Here's how the part is built. I have some questions about the finished solid (model axes, mm). A direction names the side the tool comes from. Coordinates: 2 decimals unless noted, no trailing zeros. Order: outer loops, then holes, each group sorted by start corner. A loop starts at its lowest first (then second) coordinate and runs counter-clockwise, first axis right, second up.
```python
from build123d import *

# Parameters (mm, degrees)
BOSS_EXTRUDE1_DEPTH = 6.35


with BuildPart() as part:
    # Sketch2 → Boss-Extrude1 (new body)
    with BuildSketch(Plane(origin=(0, 0, 0), x_dir=(1, 0, 0), z_dir=(0, 1, 0))):
        with BuildLine():
            Line((-50.75013925, 9.494238665), (-40.191557527, 3.398238665))
            Line((-40.191557527, 3.398238665), (-50.75013925, -2.697761335))
            Line((-50.75013925, -2.697761335), (-40.191557527, -8.793761335))
            Line((-40.191557527, -8.793761335), (-50.75013925, -14.889761335))
            Line((-50.75013925, -14.889761335), (-64.40263925, -14.889761335))
            ThreePointArc((-64.40263925, -14.889761335), (-65.584061474, -2.697761335), (-64.40263925, 9.494238665))
            Line((-64.40263925, 9.494238665), (-50.75013925, 9.494238665))
        make_face()
    extrude(amount=BOSS_EXTRUDE1_DEPTH)


solid = part.part
```
Q1. For faces 1 (the flat face through (-45.545, 3.131, 5.703)), 2 (the flat face through (-45.545, 3.131, -6.489)), which set-ups out of +Z, -Z, +X, -X, +Y, -Y let a thin tool reach every point of the face, with its end or its side?
Q2. If we section it at B-B on y = 4.5: Write out the boundary of the cut face in (x, z).
Q3. If we section it at D-D on z = 3.5: Write out the boundary of the cut face in (x, y).
Q4. We'd pull the mould along Z, two halves only. Please class faces 3 (the flat face through (-45.4, 3.13, -0.39)), 4 (the flat face through (-56, 6.35, 3)), 5 (the flat face through (-58, 3, -9.494)): pulls with the +Z half, pulls with the -Z half, needs draft (parallel to the pull), parting line crosses it, or undercut.
Q5. If we section it at A-A on x = -47: Write out the boundary of the cut face in (y, z).
Q6. I need wall thicknesses on L1, parallel to Z at x = -46, y = 2.5; L2, parallel to Z at x = -43.75, y = 1.75; L3, parallel to X at y = 2.25, z = 12.5. Which ranges of each line are inside material? Lowest first, please.
Q7. If we section it at C-C on x = -43.25: Write out the boundary of the cut face in (y, z).
Reply:
1. face 1: +X, +Y, -Y
1. face 2: -Z, +X, +Y, -Y
2. outline: (-64.4, -9.49) - (-50.75, -9.49) - (-40.19, -3.4) - (-50.75, 2.7) - (-40.19, 8.79) - (-50.75, 14.89) - (-64.4, 14.89) arc R63.5 ccw to start
3. outline: (-65.58, 0) - (-49.36, 0) - (-49.36, 6.35) - (-65.58, 6.35) - close
4. face 3: undercut
4. face 4: needs draft
4. face 5: pulls with the -Z half
5. outline: (0, -7.33) - (6.35, -7.33) - (6.35, 0.53) - (0, 0.53) - close; (0, 4.86) - (6.35, 4.86) - (6.35, 12.72) - (0, 12.72) - close
6. L1: z = -6.75 to -0.04, 5.44 to 12.15
6. L2: z = -5.45 to -1.34, 6.74 to 10.85
6. L3: x = -64.82 to -46.61
7. outline: (0, -5.16) - (6.35, -5.16) - (6.35, -1.63) - (0, -1.63) - close; (0, 7.03) - (6.35, 7.03) - (6.35, 10.56) - (0, 10.56) - close
